Here's how the part is built. I have some questions about the finished solid (model axes, mm). Round coordinates to 2 decimals unless told otherwise and drop trailing zeros. Loops run counter-clockwise (first coordinate to the right, second up) from the corner with the lowest first, then second, coordinate; pieces in that order, holes last. Notation, with made-up numbers: M 18.5,86.25 L 30.5,86.25 A5 cw 30.5,93.25 Z; hole C 57.25,86.25 d9. An arc over 180 degrees is marked long. One line per question, with ' | ' between items. Start each with the question number.
```python
from build123d import *

# Parameters (mm, degrees)
BOSS_EXTRUDE1_DEPTH = 7
BOSS_EXTRUDE2_DEPTH = 31


with BuildPart() as part:
    # Sketch2 → Boss-Extrude1 (new body)
    with BuildSketch(Plane(origin=(-7.607664395, 31.287005672, 3.337829853), x_dir=(0.971914021301819, 0.23501337979879552, 0.0123226016926005), z_dir=(-0.23501337979879552, 0.9665075330997785, 0.10311110404281207))):
        with BuildLine():
            Line((8.938687007, -72.653651109), (-5.758907082, -79.102156982))
            Line((-5.758907082, -79.102156982), (0.267733921, -92.838226224))
            ThreePointArc((0.267733921, -92.838226224), (7.833125922, -90.10764187), (14.96532801, -86.389720351))
            Line((14.96532801, -86.389720351), (8.938687007, -72.653651109))
        make_face()
    extrude(amount=-BOSS_EXTRUDE1_DEPTH)

    # Sketch4 → Boss-Extrude2 (add)
    with BuildSketch(Plane(origin=(28.173765631, 2.9e-08, 64.214343511), x_dir=(-0.9157379494904142, 6.021465183735281e-11, 0.4017760668122129), z_dir=(-0.40177606681221284, -4.1173746889623063e-10, -0.9157379494904141))):
        with BuildLine():
            Line((32.238376721, 21.932158606), (39.003929453, 20.135690895))
            ThreePointArc((39.003929453, 20.135690895), (40.42366803, 17.68939934), (37.977376475, 16.269660762))
            Line((37.977376475, 16.269660762), (31.211823744, 18.066128473))
            ThreePointArc((31.211823744, 18.066128473), (29.792085166, 20.512420028), (32.238376721, 21.932158606))
        make_face()
    extrude(amount=-BOSS_EXTRUDE2_DEPTH)


solid = part.part
```
1) I'm going to push flat-ended pins straight in: pin 1 Ø12 at (x, z) = (8.5, 100) entering from +Y; pin 2 Ø2 at (x, y) = (6.5, 20) entering from +Z; pin 3 Ø1 at (x, z) = (3.5, 97.5) entering from +Y. Where does each tip first touch, or does it pass through?
2) Imagine slicing it at A-A (z = 88). Write out the boundary of the cut face in (x, y).
3) We'd pull the mould along Z, two halves only. Please class faces 1 (the face through (-0.61, 17.05, 84.83)), 2 (the face through (4.882, 21.047, 99.669)), 3 (the face through (10.156, 20.47, 97.272)): pulls with the +Z half, pulls with the -Z half, needs draft (parallel to the pull), parting line crosses it, or undercut.
4) Please list where these lines run through material, in increasing order: L1, parallel to Y at x = -4, z = 92; L2, parallel to Y at x = -6, z = 82; L3, parallel to Z at x = -5.5, y = 17.25. Write a range as from..to.
Results are:
1) pin 1: y = 22 | pin 2: z = 108.01 | pin 3: y = 21.07
2) outline: M -9.57,21.78 L -7.61,15.01 L 9.33,19.13 L 7.37,25.9 Z
3) face 1: pulls with the -Z half | face 2: pulls with the +Z half | face 3: undercut
4) L1: 15.46..22.71 | L2: 16.04..23.29 | L3: 78.99..94.29
